Verification items for this drawing (mm, ordinates from the low corner). A direction names the side the tool comes from. Coordinates: 2 decimals unless noted, no trailing zeros. Order: outer loops, then holes, each group sorted by start corner. A loop starts at its lowest first (then second) coordinate and runs counter-clockwise, first axis right, second up.
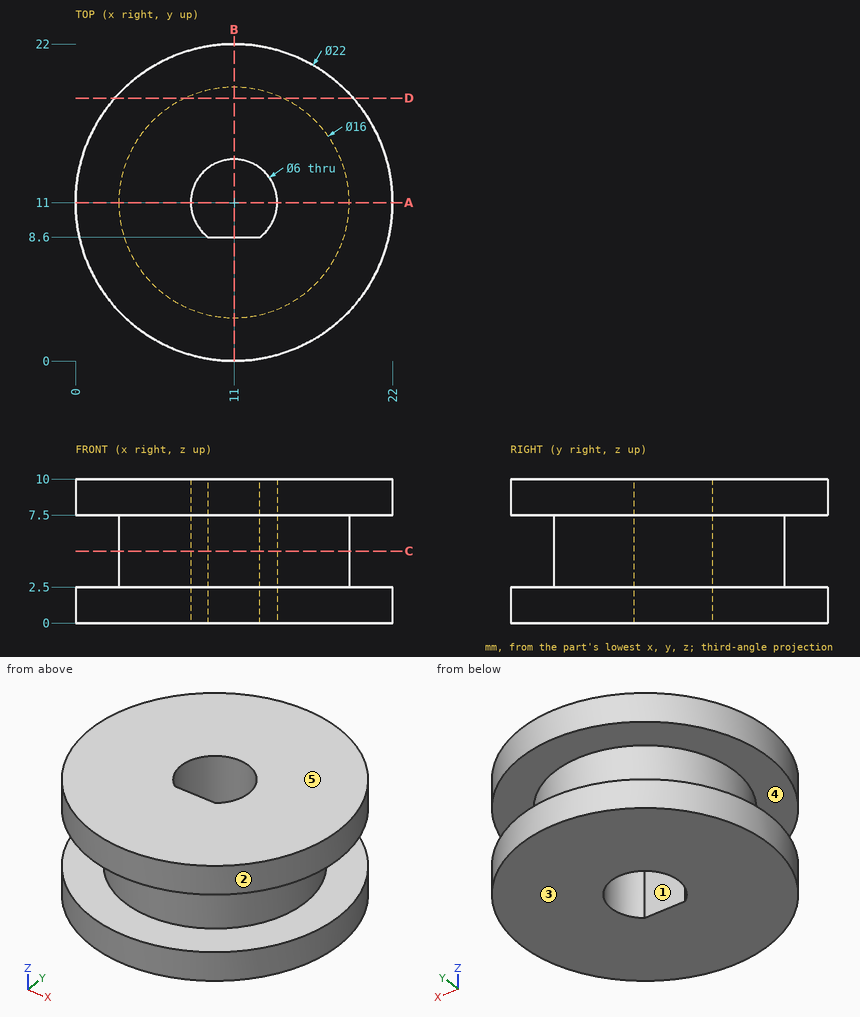
(1) Cross-section at A-A (y = 11). Enter the section's corners in (x, z).
Filled in:
outline: (0, 0) - (8, 0) - (8, 10) - (0, 10) - (0, 7.5) - (3, 7.5) - (3, 2.5) - (0, 2.5) - close; (14, 0) - (22, 0) - (22, 2.5) - (19, 2.5) - (19, 7.5) - (22, 7.5) - (22, 10) - (14, 10) - close
(2) Release check for a two-part mould opening along X. For the marked faces 1, 2 and 3 record: +X half, -X half, draft (parallel to the pull), parting line (faces both ways), or undercut.
Filled in:
face 1: undercut
face 2: parting line
face 3: draft
(3) Cross-section at B-B (x = 11). Enter the section's corners in (y, z), and give its area (3 significant figures).
Filled in:
outline: (0, 0) - (8.6, 0) - (8.6, 10) - (0, 10) - (0, 7.5) - (3, 7.5) - (3, 2.5) - (0, 2.5) - close; (14, 0) - (22, 0) - (22, 2.5) - (19, 2.5) - (19, 7.5) - (22, 7.5) - (22, 10) - (14, 10) - close
area: 136 mm2
(4) Tool access check on the marked faces 4 and 5. Record the directions out of +Z, -Z, +X, -X, +Y, -Y that give a thin tool (end or side, any length) a straight path to the whole face; none if there is none.
Filled in:
face 4: none
face 5: +Z, +X, -X, +Y, -Y
(5) Cross-section at C-C (z = 5). Enter the section's corners in (x, y).
Filled in:
outline: circle Ø16 at (11, 11); hole (9.2, 8.6) - (12.8, 8.6) arc R3 ccw (long way) to start
(6) Cross-section at D-D (y = 18.25). Enter the section's corners in (x, z), and give its area (3 significant figures).
Filled in:
outline: (2.73, 0) - (19.27, 0) - (19.27, 2.5) - (14.38, 2.5) - (14.38, 7.5) - (19.27, 7.5) - (19.27, 10) - (2.73, 10) - (2.73, 7.5) - (7.62, 7.5) - (7.62, 2.5) - (2.73, 2.5) - close
area: 117 mm2
(7) Go/stop test with flat-tipped pins: P1, Ø4, axis at x = 3.5, z = 4, coming from the -Y side; P2, Ø2, axis at x = 12.5, z = 7, coming from the -Y side; P3, Ø11, axis at x = 12, y = 9.5, coming from the -Z side; P4, Ø1, axis at y = 3, z = 8.5, coming from the -X side. Record where each tip stops, or that it passes through.
Filled in:
P1: stops at y = 1.9
P2: stops at y = 0.02
P3: stops at z = 0
P4: stops at x = 2.95
(8) Thickness scan on probe 1 along Y at (x, z) = (11, 3); probe 2 along X at (y, z) = (11, 6.25); probe 3 along Z at (x, y) = (12.25, 19). Record the ranges inside material, lowest first.
Filled in:
probe 1: y = 3 to 8.6, 14 to 19
probe 2: x = 3 to 8, 14 to 19
probe 3: z = 0 to 2.5, 7.5 to 10
